Source: CAD feature listing. Evaluate the final solid. Frame: model axes, mm. A direction names the side the tool comes from. Round coordinates to 2 decimals unless told otherwise and drop trailing zeros. Order: outer loops, then holes, each group sorted by start corner. A loop starts at its lowest first (then second) coordinate and runs counter-clockwise, first axis right, second up. Notation, with made-up numbers: M 12,38.25 L 35,38.25 A22 cw 35,69.25 Z; hole C 20.25,-2.5 d11. An arc over 180 degrees is marked long. Answer as CSV lines item,"result". Start each with the question number.
Item 1: Set-up query: faces 4 (the face through (-10.25, 20, 4)), 5 (the face through (-10.25, -20, 4)), 6 (the face through (18.439, 19, 4)), 7 (the face through (-18.439, 19, 4)). Return all of +Z, -Z, +X, -X, +Y, -Y with unobstructed straight access to the full face (end or side cutting, diameter ignored); none if empty.
Item 2: Section query D-D on y = 10. Return the cut outline in (x, z), plus the area to 3 significant figures.
Item 3: First-contact query: P1, Ø2.5, axis at y = 21.5, z = 6, coming from the +X side; P2, Ø4.5, axis at y = -20, z = 4, coming from the -X side; P3, Ø1, axis at y = -1.5, z = 2, coming from the -X side. Flat tips, straight axial feed; report the tip coordinate or a pass-through.
Item 4: Section query A-A on y = -22. Return the cut outline in (x, z), plus the area to 3 significant figures.
Item 5: Line query: line 1 (X direction, y = 20.5, z = 5.5); line 2 (Z direction, x = 16.25, y = 22); line 3 (Y direction, x = 12, z = 4.25). Output: solid intervals per line, ascending. Write a range as [from, to].
Item 6: Section query B-B on x = 17.5. Return the cut outline in (y, z).
Item 7: Pull-direction query (X, two-part tool) for faces 1 (the face through (-14, -25, 1)), 2 (the face through (-13.34, -15.57, 4.56)), 3 (the face through (22, 0, 4)); classes: +X half, -X half, draft (parallel to the pull), parting line (faces both ways), or undercut.
Item 8: Section query C-C on z = 1. Return the cut outline in (x, y), plus the area to 3 significant figures.
from build123d import *

# Parameters (mm, degrees)
F1_DEPTH = 9
F2_D     = 3.2
F2_DEPTH = 9
F4_D     = 3.2
F4_DEPTH = 40
F5_SIZE  = 2


with BuildPart() as f1:
    # F0 (on Top) → F1 (new body)
    with BuildSketch(Plane.XY):
        with BuildLine():
            Line((18.439089, -12), (10.957304, -12))
            ThreePointArc((10.957304, -12), (0, -16.25), (-10.957304, -12))
            Line((-10.957304, -12), (-18.439089, -12))
            Line((-18.439089, -12), (-18.439089, -26))
            Line((-18.439089, -26), (-10.25, -26))
            Line((-10.25, -26), (-10.25, -18))
            Line((-10.25, -18), (10.25, -18))
            Line((10.25, -18), (10.25, -26))
            Line((10.25, -26), (18.439089, -26))
            Line((18.439089, -26), (18.439089, -12))
        make_face()
        with BuildLine():
            ThreePointArc((-10.957304, -12), (-16.25, 0), (-10.957304, 12))
            Line((-10.957304, 12), (-18.439089, 12))
            ThreePointArc((-18.439089, 12), (-22, 0), (-18.439089, -12))
            Line((-18.439089, -12), (-10.957304, -12))
        make_face()
        with BuildLine():
            ThreePointArc((-10.957304, 12), (0, 16.25), (10.957304, 12))
            Line((10.957304, 12), (18.439089, 12))
            Line((18.439089, 12), (18.439089, 26))
            Line((18.439089, 26), (10.25, 26))
            Line((10.25, 26), (10.25, 18))
            Line((10.25, 18), (-10.25, 18))
            Line((-10.25, 18), (-10.25, 26))
            Line((-10.25, 26), (-18.439089, 26))
            Line((-18.439089, 26), (-18.439089, 12))
            Line((-18.439089, 12), (-10.957304, 12))
        make_face()
        with BuildLine():
            ThreePointArc((10.957304, 12), (14.868064, 6.557679), (16.25, 0))
            ThreePointArc((16.25, 0), (14.868064, -6.557679), (10.957304, -12))
            Line((10.957304, -12), (18.439089, -12))
            ThreePointArc((18.439089, -12), (22, 0), (18.439089, 12))
            Line((18.439089, 12), (10.957304, 12))
        make_face()
    extrude(amount=F1_DEPTH)

    # F2
    with Locations(Plane(origin=(0, 0, 0), x_dir=(1, 0, 0), z_dir=(0, 0, -1))):
        with Locations((-14.939089, -15.5), (14.939089, -15.5), (14.939089, 15.5), (-14.939089, 15.5)):
            Hole(F2_D / 2, depth=F2_DEPTH)

    # F4
    with Locations(Plane.YZ.offset(18.439089)):
        with Locations((-22, 4.5), (22, 4.5)):
            Hole(F4_D / 2, depth=F4_DEPTH)

    # F5
    f5_edges = [f1.edges().sort_by_distance(p)[0] for p in [
        (14.344544, 26, 9),
        (14.344544, 26, 0),
        (-14.344544, 26, 9),
        (-14.344544, 26, 0),
        (-14.344544, -26, 9),
        (14.344544, -26, 9),
        (14.344544, -26, 0),
        (-14.344544, -26, 0),
    ]]
    chamfer(f5_edges, length=F5_SIZE)


solid = f1.part
Results:
1,face 4,"+Z, -Z, +Y"
1,face 5,"+Z, -Z, -Y"
1,face 6,"+Z, -Z, +X, +Y"
1,face 7,"+Z, -Z, -X, +Y"
2,outline,"M -19.6,0 L -12.81,0 L -12.81,9 L -19.6,9 Z; M 12.81,0 L 19.6,0 L 19.6,9 L 12.81,9 Z"
2,area,"122 mm^2"
3,P1,"x = 18.44"
3,P2,"x = -18.44"
3,P3,"x = -21.98"
4,outline,"M -18.44,0 L -10.25,0 L -10.25,2.9 L -18.44,2.9 Z; M -18.44,6.1 L -10.25,6.1 L -10.25,9 L -18.44,9 Z; M 10.25,0 L 18.44,0 L 18.44,2.9 L 10.25,2.9 Z; M 10.25,6.1 L 18.44,6.1 L 18.44,9 L 10.25,9 Z"
4,area,"95.0 mm^2"
5,line 1,"[-18.44, -10.25], [10.25, 18.44]"
5,line 2,"[0, 2.9], [6.1, 9]"
5,line 3,"[-26, -23.58], [-20.42, -10.96], [10.96, 20.42], [23.58, 26]"
6,outline,"M -26,2 L -24,0 L 24,0 L 26,2 L 26,7 L 24,9 L -24,9 L -26,7 Z; hole C -22,4.5 d3.2; hole C 22,4.5 d3.2"
7,face 1,"draft"
7,face 2,"undercut"
7,face 3,"+X half"
8,outline,"M -18.44,-25 L -10.25,-25 L -10.25,-18 L 10.25,-18 L 10.25,-25 L 18.44,-25 L 18.44,-12 A22 ccw 18.44,12 L 18.44,25 L 10.25,25 L 10.25,18 L -10.25,18 L -10.25,25 L -18.44,25 L -18.44,12 A22 ccw -18.44,-12 Z; hole C -14.94,-15.5 d3.2; hole C -14.94,15.5 d3.2; hole M -10.96,-12 A16.25 ccw 10.96,-12 A16.25 ccw 16.25,0 A16.25 ccw 10.96,12 A16.25 ccw -10.96,12 A16.25 ccw Z; hole C 14.94,-15.5 d3.2; hole C 14.94,15.5 d3.2"
8,area,"811 mm^2"
